```python
from build123d import *

# Parameters (mm, degrees)
F0_R     = 6.5
F0_R_2   = 5
F1_DEPTH = 6
F2_R     = 5.761046585
F2_R_2   = 5
F3_DEPTH = 1
F4_R     = 6.5
F4_R_2   = 5
F5_DEPTH = 3.05
F6_R     = 5.693586081
F6_R_2   = 5
F7_DEPTH = 1
F8_R     = 6.5
F8_R_2   = 5
F9_DEPTH = 1


with BuildPart() as f1:
    # F0 (on Front) → F1 (new body)
    with BuildSketch(Plane.XZ):
        Circle(F0_R)
        Circle(F0_R_2, mode=Mode.SUBTRACT)
    extrude(amount=F1_DEPTH)

    # F2 (on face) → F3 (join)
    with BuildSketch(Plane.XZ.offset(6)):
        Circle(F2_R)
        Circle(F2_R_2, mode=Mode.SUBTRACT)
    extrude(amount=F3_DEPTH)

    # F4 (on face) → F5 (join)
    with BuildSketch(Plane.XZ.offset(7)):
        Circle(F4_R)
        Circle(F4_R_2, mode=Mode.SUBTRACT)
    extrude(amount=F5_DEPTH)

    # F6 (on face) → F7 (join)
    with BuildSketch(Plane.XZ.offset(10.05)):
        Circle(F6_R)
        Circle(F6_R_2, mode=Mode.SUBTRACT)
    extrude(amount=F7_DEPTH)

    # F8 (on face) → F9 (join)
    with BuildSketch(Plane.XZ.offset(11.05)):
        Circle(F8_R)
        Circle(F8_R_2, mode=Mode.SUBTRACT)
    extrude(amount=F9_DEPTH)


solid = f1.part
```
Source: CAD feature listing. Evaluate the final solid. Frame: model axes, mm. A direction names the side the tool comes from. Coordinates: 2 decimals unless noted, no trailing zeros. Write each loop counter-clockwise with the first axis right and the second up, starting at its lowest first coordinate (ties: lowest second). Pieces come first, ordered by that corner, then holes. Notation, with made-up numbers: (87, 33.25) -> (91, 33.25) arc R35 ccw to (91, 72.25) -> close; hole circle Ø3 at (39.25, -28.5). An arc over 180 degrees is marked (long way). Return JSON: item names as keys, results as strings. Group by question number.
1) Section query C-C, the plane y = -9.25. Return loops of the section in (x, z), plus the area to 3 significant figures.
2) Section query A-A, the plane z = 0. Return loops of the section in (x, y), plus the area to 3 significant figures.
3) Mould query, pull axis Z, two halves, no side actions, for faces 3 (the face through (-1, -7, -6)), 4 (the face through (-1.08, -5.94, -4.88)), 5 (the face through (-5.158, -8.504, -3.955)). Classes: +Z half, -Z half, draft (parallel to the pull), parting line (faces both ways), or undercut.
4) Section query B-B, the plane x = 0. Return loops of the section in (y, z), plus the area to 3 significant figures.
5) Contact query for flat-ended pins moving along their axis: P1, Ø2, axis at y = -4.5, z = -2.5, coming from the -X side; P2, Ø2, axis at y = -4.5, z = 3, coming from the +X side; P3, Ø3, axis at y = -6.5, z = -4.5, coming from the +X side. Output: stop coordinate, or through.
6) Set-up query: faces 1 (the face through (0, -11.05, -6)), 2 (the face through (2, -12.05, -5)). Return all of +Z, -Z, +X, -X, +Y, -Y with unobstructed straight access to the full face (end or side cutting, diameter ignored); none if empty.
7) Ray query, line 1 along Y through (x, z) = (5, -3.75); line 2 along Z through (x, y) = (0, -3); line 3 along Z through (x, y) = (2, -8.25). Return the intervals inside material, ascending.
From the geometry:
{
 "1": {"outline": "circle Ø13 at (0, 0); hole circle Ø10 at (0, 0)", "area": "54.2 mm²"},
 "2": {"outline": "(-6.5, -12.05) -> (-5, -12.05) -> (-5, 0) -> (-6.5, 0) -> (-6.5, -6) -> (-5.76, -6) -> (-5.76, -7) -> (-6.5, -7) -> (-6.5, -10.05) -> (-5.69, -10.05) -> (-5.69, -11.05) -> (-6.5, -11.05) -> close; (5, -12.05) -> (6.5, -12.05) -> (6.5, -11.05) -> (5.69, -11.05) -> (5.69, -10.05) -> (6.5, -10.05) -> (6.5, -7) -> (5.76, -7) -> (5.76, -6) -> (6.5, -6) -> (6.5, 0) -> (5, 0) -> close", "area": "33.1 mm²"},
 "3": {"face 3": "draft", "face 4": "undercut", "face 5": "parting line"},
 "4": {"outline": "(-12.05, -6.5) -> (-11.05, -6.5) -> (-11.05, -5.69) -> (-10.05, -5.69) -> (-10.05, -6.5) -> (-7, -6.5) -> (-7, -5.76) -> (-6, -5.76) -> (-6, -6.5) -> (0, -6.5) -> (0, -5) -> (-12.05, -5) -> close; (-12.05, 5) -> (0, 5) -> (0, 6.5) -> (-6, 6.5) -> (-6, 5.76) -> (-7, 5.76) -> (-7, 6.5) -> (-10.05, 6.5) -> (-10.05, 5.69) -> (-11.05, 5.69) -> (-11.05, 6.5) -> (-12.05, 6.5) -> close", "area": "33.1 mm²"},
 "5": {"P1": "x = -6.32", "P2": "x = 6.18", "P3": "x = 5.72"},
 "6": {"face 1": "none", "face 2": "+Z, -Z, +X, -X, -Y"},
 "7": {"line 1": "-12.05 to -11.05, -10.05 to -7, -6 to 0", "line 2": "-6.5 to -5, 5 to 6.5", "line 3": "-6.18 to -4.58, 4.58 to 6.18"}
}
